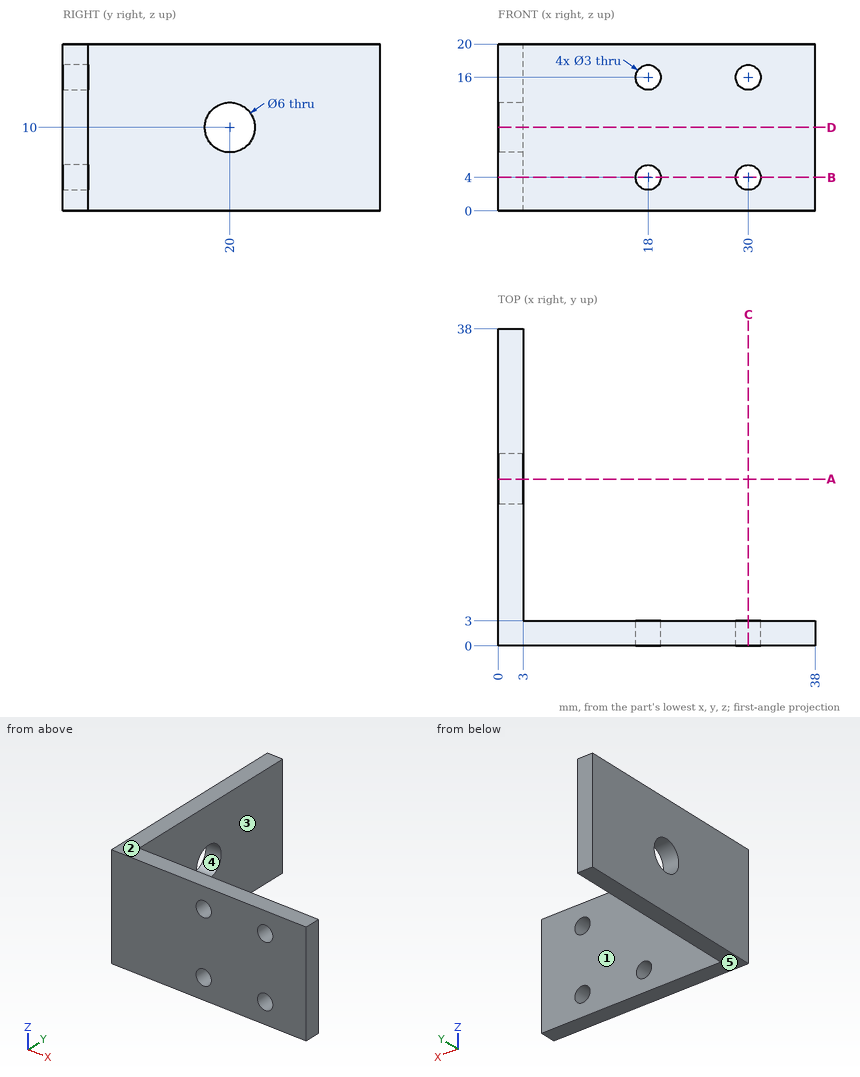
Input: dimensioned drawing with shaded views. Units: mm. Origin: part minimum x, y, z. A direction names the side the tool comes from. Give positions to 0.01 mm unless a question says otherwise; leave off trailing zeros. Write each loop counter-clockwise with the first axis right and the second up, starting at its lowest first coordinate (ties: lowest second). Pieces come first, ordered by that corner, then holes.
1. Section query D-D (z = 10). Return the cut outline in (x, y).
2. Material intervals for line 1 along X through (y, z) = (0.95, 16); line 2 along Y through (x, z) = (1.2, 10); line 3 along Y through (x, z) = (8.5, 18.5), sorted ascending.
3. Pull-direction query (Z, two-part tool) for the marked faces 3, 4 and 5; classes: +Z half, -Z half, draft (parallel to the pull), parting line (faces both ways), or undercut.
4. Section query B-B (z = 4). Return the cut outline in (x, y), then the cut area to 3 significant figures.
5. Section query C-C (x = 30). Return the cut outline in (y, z), then the cut area to 3 significant figures.
6. Section query A-A (y = 20). Return the cut outline in (x, z), then the cut area to 3 significant figures.
7. Access query for the marked faces 1 and 2. Directions: +Z, -Z, +X, -X, +Y, -Y. A direction counts if a zero-diameter tool reaches every point of the face in a straight line with its end or side. Return the directions, or none.
8. First-contact query: pin 1 (3.5 mm diameter, centred on x = 30, z = 4, fed in from +Y); pin 2 (5 mm diameter, centred on x = 7, z = 17.5, fed in from -Y); pin 3 (4 mm diameter, centred on y = 18, z = 6.5, fed in from +X); pin 4 (2.5 mm diameter, centred on x = 18, z = 16, fed in from +Y). Flat tips, straight axial feed; report the tip coordinate or a pass-through.
Output values:
1. outline: (0, 0) - (38, 0) - (38, 3) - (3, 3) - (3, 17) - (0, 17) - close; (0, 23) - (3, 23) - (3, 38) - (0, 38) - close
2. line 1: x = 0 to 16.5, 19.5 to 28.5, 31.5 to 38
2. line 2: y = 0 to 17, 23 to 38
2. line 3: y = 0 to 3
3. face 3: draft
3. face 4: undercut
3. face 5: -Z half
4. outline: (0, 0) - (16.5, 0) - (16.5, 3) - (3, 3) - (3, 38) - (0, 38) - close; (19.5, 0) - (28.5, 0) - (28.5, 3) - (19.5, 3) - close; (31.5, 0) - (38, 0) - (38, 3) - (31.5, 3) - close
4. area: 201 mm2
5. outline: (0, 0) - (3, 0) - (3, 2.5) - (0, 2.5) - close; (0, 5.5) - (3, 5.5) - (3, 14.5) - (0, 14.5) - close; (0, 17.5) - (3, 17.5) - (3, 20) - (0, 20) - close
5. area: 42.0 mm2
6. outline: (0, 0) - (3, 0) - (3, 7) - (0, 7) - close; (0, 13) - (3, 13) - (3, 20) - (0, 20) - close
6. area: 42.0 mm2
7. face 1: +Z, -Z, +X, +Y
7. face 2: +Z, +X, -X, +Y, -Y
8. pin 1: stops at y = 3
8. pin 2: stops at y = 0
8. pin 3: stops at x = 3
8. pin 4: passes through
